Geometry: final body of the model. Coordinates: model frame, mm. Face numbers are marked on the shaded views. A direction names the side the tool comes from. Give positions to 0.01 mm unless a question says otherwise; leave off trailing zeros. Loops run counter-clockwise (first coordinate to the right, second up) from the corner with the lowest first, then second, coordinate; pieces in that order, holes last. Notation, with made-up numbers: (78, 73.5) - (129, 73.5) arc R22 ccw to (129, 87.5) - close; hole circle Ø5 at (-1, 68.25). An arc over 180 degrees is marked (long way). Use one line per item in the form item = value.
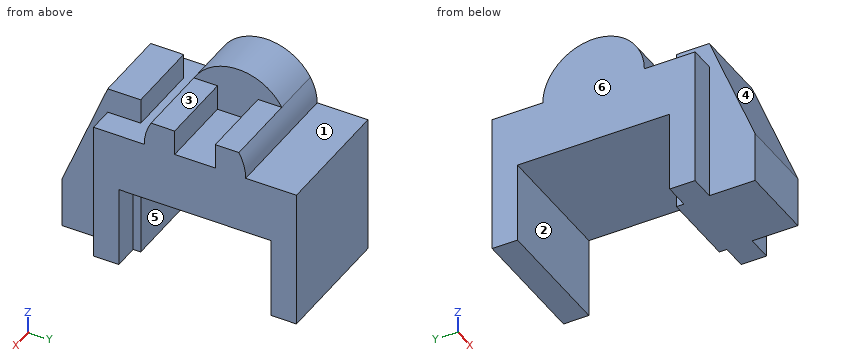
```python
from build123d import *

# Parameters (mm, degrees)
F1_DEPTH      = 25
F2_W          = 30
F2_H          = 65
F3_DEPTH      = 18
F3_DEPTH_BACK = 13
F4_SIZE2      = 18
F4_SIZE       = 45
F6_DEPTH      = 20


with BuildPart() as f1:
    # F0 (on Right) → F1 (new body, symmetric)
    with BuildSketch(Plane.YZ):
        with BuildLine():
            Line((8, 0), (0, 0))
            Line((0, 0), (-8, 0))
            Line((-8, 0), (-8, 10))
            Line((-8, 10), (-17.3205080757, 10))
            ThreePointArc((-17.3205080757, 10), (-19.3185165258, 5.1763809021), (-20, 0))
            Line((-20, 0), (-40, 0))
            Line((-40, 0), (-40, -55))
            Line((-40, -55), (-30, -55))
            Line((-30, -55), (-30, -23))
            Line((-30, -23), (0, -23))
            Line((0, -23), (30, -23))
            Line((30, -23), (30, -55))
            Line((30, -55), (40, -55))
            Line((40, -55), (40, 0))
            Line((40, 0), (20, 0))
            ThreePointArc((20, 0), (19.3185165258, 5.1763809021), (17.3205080757, 10))
            Line((17.3205080757, 10), (8, 10))
            Line((8, 10), (8, 0))
        make_face()
    extrude(amount=F1_DEPTH, both=True)

    # F2 (on face) → F3 (join, two sides)
    with BuildSketch(Plane.XZ.offset(40)) as f3_sk:
        with Locations((0, -22.5)):
            Rectangle(F2_W, F2_H)
    extrude(amount=F3_DEPTH)
    extrude(f3_sk.sketch, amount=-F3_DEPTH_BACK)

    # F4
    f4_edges = [f1.edges().sort_by_distance(p)[0] for p in [
        (0, -58, 10),
    ]]
    f4_side = f1.faces().sort_by_distance((0, -58, -22.5))[0]
    chamfer(f4_edges, length=F4_SIZE, length2=F4_SIZE2, reference=f4_side)

    # F5 (on face) → F6 (join)
    with BuildSketch(Plane(origin=(-25, 0, 0), x_dir=(0, -1, 0), z_dir=(-1, 0, 0))):
        with BuildLine():
            Line((-20, 0), (20, 0))
            ThreePointArc((20, 0), (0, 20), (-20, 0))
        make_face()
    extrude(amount=-F6_DEPTH)


solid = f1.part
```
(1) Cut plane C-C (z = -20). Return the cut outline in (x, y).
Solution:
outline = (-25, -40) - (-15, -40) - (-15, -52) - (15, -52) - (15, -40) - (25, -40) - (25, 40) - (-25, 40) - close
(2) Cut plane B-B (x = 18.5). Return the cut outline in (y, z), plus the area to 3 significant figures.
Solution:
outline = (-40, -55) - (-30, -55) - (-30, -23) - (30, -23) - (30, -55) - (40, -55) - (40, 0) - (20, 0) arc R20 ccw to (17.32, 10) - (8, 10) - (8, 0) - (-8, 0) - (-8, 10) - (-17.32, 10) arc R20 ccw to (-20, 0) - (-40, 0) - close
area = 2,700 mm2
(3) Access query for the marked faces 1, 2 and 3. Directions: +Z, -Z, +X, -X, +Y, -Y. A direction counts if a zero-diameter tool reaches every point of the face in a straight line with its end or side. Return the directions, or none.
Solution:
face_1 = +Z, +X, -X, +Y
face_2 = -Z, +X, -X
face_3 = +Z, +X, +Y, -Y
(4) Pull-direction query (Y, two-part tool) for the marked faces 4, 5 and 6; classes: released by +Y, released by -Y, zero draft, split by the parting line, or undercut.
Solution:
face_4 = released by -Y
face_5 = undercut
face_6 = zero draft
(5) Pin query (flat end, axial travel): P1, Ø6, axis at x = 0.5, y = 11, coming from the +Z side; P2, Ø3, axis at x = 5, z = 6.5, coming from the +Y side; P3, Ø5, axis at x = 15.5, y = 4, coming from the +Z side. Return the tip coordinate at first contact, or that it passes through.
Solution:
P1 = 10
P2 = 19.36
P3 = 0
(6) Cut plane A-A (z = -48.5). Return the cut outline in (x, y), plus the area to 3 significant figures.
Solution:
outline = (-25, -40) - (-15, -40) - (-15, -58) - (15, -58) - (15, -40) - (25, -40) - (25, -30) - (15, -30) - (15, -27) - (-15, -27) - (-15, -30) - (-25, -30) - close; (-25, 30) - (25, 30) - (25, 40) - (-25, 40) - close
area = 1,630 mm2
(7) Cut plane D-D (y = 26). Return the cut outline in (x, z), plus the area to 3 significant figures.
Solution:
outline = (-25, -23) - (25, -23) - (25, 0) - (-25, 0) - close
area = 1,150 mm2
(8) Material intervals for L1, parallel to Y at x = 20, z = -33; L2, parallel to Y at x = -5.5, z = -40.5; L3, parallel to Z at x = 13, y = -15.5, sorted ascending. Write a range as from..to.
Solution:
L1 = -40..-30, 30..40
L2 = -58..-27, 30..40
L3 = -23..10
